Source: three-view drawing plus pictorial views. Frame: mm from the lowest corner of the part. A direction names the side the tool comes from. Round coordinates to 2 decimals unless told otherwise and drop trailing zeros. Loops run counter-clockwise (first coordinate to the right, second up) from the corner with the lowest first, then second, coordinate; pieces in that order, holes last. Notation, with made-up numbers: (51, -12) -> (100, -12) arc R37 cw to (100, 26) -> close; hole circle Ø10 at (-39.5, 24). An arc over 180 degrees is marked (long way). Answer in a Markdown table with one row per item. Add a question column.
Q1. Section A-A, the plane x = 10.5. Output: boundary loops of the cut face in (y, z).
Q2. Section C-C, the plane z = 7.5. Output: boundary loops of the cut face in (x, y), and give its area (3 significant figures).
Q3. Section D-D, the plane y = 3.6. Output: boundary loops of the cut face in (x, z), and give its area (3 significant figures).
Q4. Section B-B, the plane z = 2.5. Output: boundary loops of the cut face in (x, y), and give its area (3 significant figures).
Q5. Reachability of the marked faces 1 and 2 from +Z, -Z, +X, -X, +Y, -Y: full face, straight path, thin tool, end or side. Return the list, or none.
Q6. Mould query, pull axis X, two halves, no side actions, for the marked faces 3, 4 and 5. Classes: pulls with the +X half, pulls with the -X half, needs draft (parallel to the pull), parting line crosses it, or undercut.
Q7. Pin query (flat end, axial travel): pin 1 (2.5 mm diameter, centred on x = 10.5, z = 2.5, fed in from -Y); pin 2 (3 mm diameter, centred on y = 2, z = 3.5, fed in from -X); pin 3 (5 mm diameter, centred on x = 6.5, z = 4.5, fed in from -Y); pin 4 (0.8 mm diameter, centred on y = 4.5, z = 7, fed in from +X). Return the tip coordinate at first contact, or that it passes through.
Q8. Ray query, L1, parallel to X at y = 2.95, z = 2.5; L2, parallel to Z at x = 10.5, y = 3.25; L3, parallel to X at y = 1, z = 7.25. Return the intervals inside material, ascending. Write a range as from..to.
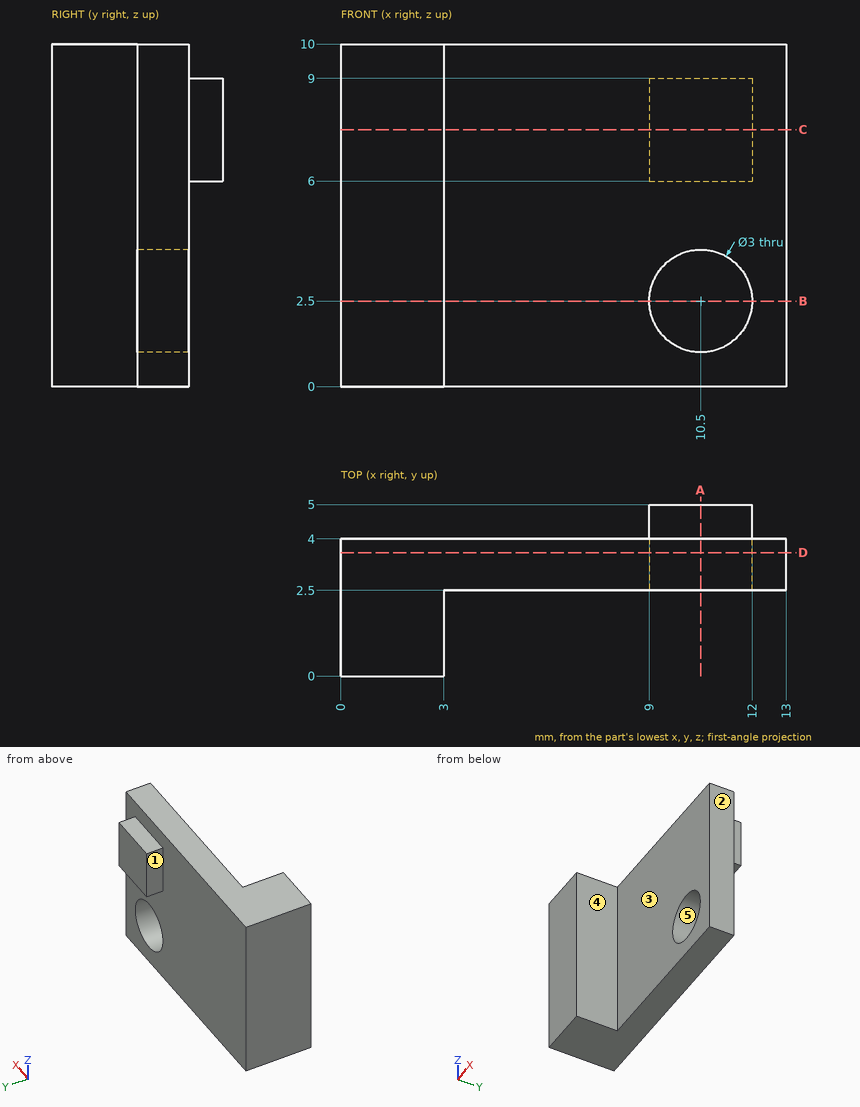
Answer block:
| question | item | result |
|---|---|---|
| 1 | outline | (2.5, 0) -> (4, 0) -> (4, 1) -> (2.5, 1) -> close; (2.5, 4) -> (4, 4) -> (4, 6) -> (5, 6) -> (5, 9) -> (4, 9) -> (4, 10) -> (2.5, 10) -> close |
| 2 | outline | (0, 0) -> (3, 0) -> (3, 2.5) -> (13, 2.5) -> (13, 4) -> (12, 4) -> (12, 5) -> (9, 5) -> (9, 4) -> (0, 4) -> close |
| 2 | area | 30.0 mm^2 |
| 3 | outline | (0, 0) -> (13, 0) -> (13, 10) -> (0, 10) -> close; hole circle Ø3 at (10.5, 2.5) |
| 3 | area | 123 mm^2 |
| 4 | outline | (0, 0) -> (3, 0) -> (3, 2.5) -> (9, 2.5) -> (9, 4) -> (0, 4) -> close; (12, 2.5) -> (13, 2.5) -> (13, 4) -> (12, 4) -> close |
| 4 | area | 22.5 mm^2 |
| 5 | face 1 | +Z, -Z, -X, +Y |
| 5 | face 2 | +Z, -Z, +X, +Y, -Y |
| 6 | face 3 | needs draft |
| 6 | face 4 | pulls with the +X half |
| 6 | face 5 | undercut |
| 7 | pin 1 | through |
| 7 | pin 2 | x = 0 |
| 7 | pin 3 | y = 2.5 |
| 7 | pin 4 | x = 12 |
| 8 | L1 | 0..9, 12..13 |
| 8 | L2 | 0..1, 4..10 |
| 8 | L3 | 0..3 |
